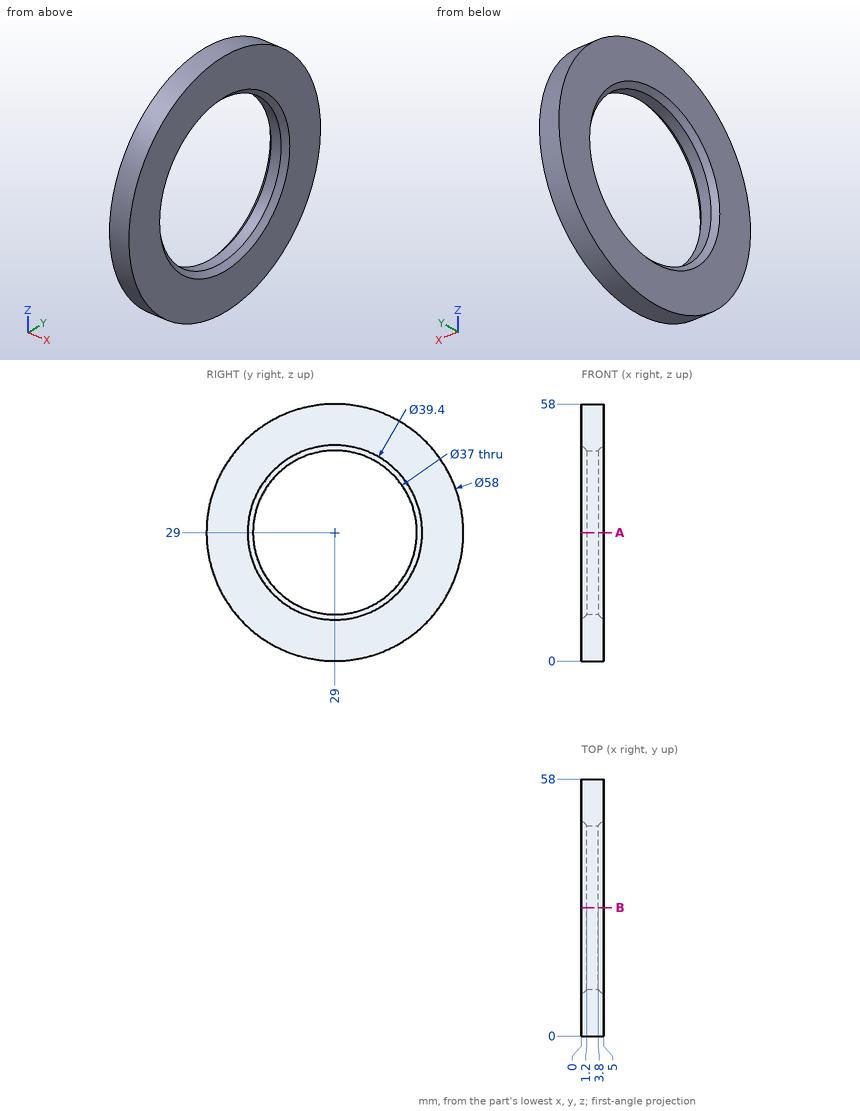
Drawing for the job (mm, zero at the part's lowest x, y, z). Give positions to 0.01 mm unless a question says otherwise; leave off trailing zeros. Order: outer loops, then holes, each group sorted by start corner. A loop starts at its lowest first (then second) coordinate and runs counter-clockwise, first axis right, second up. Notation, with made-up numbers: (-19.5, -13.75) -> (18.5, -13.75) arc R23 cw to (18.5, 8.25) -> close; hole circle Ø11 at (62, 24). An arc over 180 degrees is marked (long way). Use one line per item in the form item = value.
(1) Saw through at A-A (z = 29). Write the cut outline in (x, y).
Solution:
outline = (0, 0) -> (5, 0) -> (5, 9.3) -> (3.8, 10.5) -> (1.2, 10.5) -> (0, 9.3) -> close; (0, 48.7) -> (1.2, 47.5) -> (3.8, 47.5) -> (5, 48.7) -> (5, 58) -> (0, 58) -> close
(2) Drill centre lines: line 1 (Y direction, x = 1.85, z = 29); line 2 (Y direction, x = 1.4, z = 41.5); line 3 (Z direction, x = 1.4, y = 25.5). Where is each one in solid material? Low to high. Write a range as from..to.
Solution:
line_1 = 0..10.5, 47.5..58
line_2 = 2.83..15.36, 42.64..55.17
line_3 = 0.21..10.83, 47.17..57.79
(3) Flat gauge pin, fed straight in: P1, Ø1.5, axis at x = 4.5, z = 40.5, coming from the -Y side. Where does the tip first touch, or does it go through?
Solution:
P1 = 2.07
